Could you check a few things on this model? Use its own coordinates, in mm. A direction names the side the tool comes from. Coordinates: 2 decimals unless noted, no trailing zeros. Write each loop counter-clockwise with the first axis right and the second up, starting at its lowest first coordinate (ties: lowest second). Pieces come first, ordered by that corner, then holes.
Autodesk Inventor part; units mm, degrees
ref_plane "s1_XY" through (10.3124, 0, 0) normal (0, 0, 1) x (1, 0, 0)
ref_plane "s1_YZ" through (10.3124, 0, 0) normal (1, 0, 0) x (0, 1, 0)
ref_plane "s1_ZX" through (10.3124, 0, 0) normal (0, 1, 0) x (0, 0, 1)
sketch "Sketch_2" plane through (0, 0, 0) normal (0, 0, 1) x (1, 0, 0)
  line L0 (12.7, 0) -> (0, 0)
  line L1 (0, 0) -> (0, 7.098)
  line L2 (0, 7.098) -> (0.8395, 7.9375)
  line L3 (0.8395, 7.9375) -> (6.6726, 7.9375)
  line L4 (6.6726, 7.9375) -> (7.5121, 7.098)
  line L5 (7.5121, 7.098) -> (7.542, 7.0708)
  arc A0 (7.542, 7.0708) -> (8.1407, 6.839) centre (8.1407, 7.7279) ccw
  line L6 (8.1407, 6.839) -> (9.4234, 6.839)
  arc A1 (9.4234, 6.839) -> (10.3124, 7.7279) centre (9.4234, 7.7279) ccw
  line L7 (10.3124, 7.7279) -> (10.3124, 7.9057)
  line L8 (10.3124, 7.9057) -> (12.7, 7.9057)
  line L9 (12.7, 7.9057) -> (12.7, 0)
  line L10 (12.7, 0) -> (0, 0)
revolve "Revolution1" add sketch "Sketch_2" angle 360 about axis through (12.7, 0, 0) along (1, 0, 0)
thread "Thread1"
sketch "Sketch_3" plane through (0, 0, 0) normal (0, 0, 1) x (1, 0, 0)
  line L0 (41.275, 0) -> (12.7, 0)
  line L1 (12.7, 0) -> (12.7, 13.3731)
  line L2 (12.7, 13.3731) -> (13.462, 14.1351)
  line L3 (13.462, 14.1351) -> (34.8615, 14.1351)
  line L4 (34.8615, 14.1351) -> (34.8615, 12.846)
  line L5 (34.8615, 12.846) -> (35.6235, 12.846)
  line L6 (35.6235, 12.846) -> (36.3855, 13.6081)
  line L7 (36.3855, 13.6081) -> (40.513, 13.6081)
  line L8 (40.513, 13.6081) -> (41.275, 12.846)
  line L9 (41.275, 12.846) -> (41.275, 0)
  line L10 (41.275, 0) -> (12.7, 0)
revolve "Revolution2" add sketch "Sketch_3" angle 360 about axis through (41.275, 0, 0) along (1, 0, 0)
sketch "Sketch_5" plane through (0, 0, 0) normal (0, 0, 1) x (1, 0, 0)
  line L0 (41.275, 0) -> (0, 0)
  line L1 (0, 0) -> (0, 4.7752)
  line L2 (0, 4.7752) -> (0.762, 4.0132)
  line L3 (0.762, 4.0132) -> (41.275, 4.0132)
  line L4 (41.275, 4.0132) -> (41.275, 0)
  line L5 (41.275, 0) -> (0, 0)
revolve "Revolution3" cut sketch "Sketch_5" angle 360 about axis through (41.275, 0, 0) along (1, 0, 0)
sketch "Sketch_40" plane through (0, 0, 0) normal (0, 1, 0) x (-1, 0, 0)
  line L0 (-27.0002, 14.1351) -> (-27.0002, 0)
  line L1 (-27.0002, 0) -> (-30.1752, 0)
  line L2 (-30.1752, 0) -> (-30.1752, 3.8208)
  line L3 (-30.1752, 3.8208) -> (-31.5423, 4.6101)
  line L4 (-31.5423, 4.6101) -> (-31.8199, 13.5001)
  line L5 (-31.8199, 13.5001) -> (-32.4549, 14.1351)
  line L6 (-32.4549, 14.1351) -> (-27.0002, 14.1351)
  line L7 (-27.0002, 14.1351) -> (-27.0002, 0)
revolve "Revolution4" cut sketch "Sketch_40" angle 360 about axis through (27.0002, 0, 14.1351) along (0, 0, 1)
sketch "Sketch_47" plane through (0, 0, 0) normal (0, 0, 1) x (1, 0, 0)
  line L0 (35.6235, 0) -> (34.8615, 0)
  line L1 (34.8615, 12.5921) -> (35.6235, 12.5921)
  line L2 (35.6235, 12.5921) -> (35.6235, 12.846)
  line L3 (35.6235, 12.846) -> (35.2425, 12.846)
  line L4 (35.2425, 12.846) -> (34.984, 13.1046)
  arc A0 (34.984, 13.2842) -> (34.984, 13.1046) centre (35.0738, 13.1944) ccw
  line L5 (34.984, 13.2842) -> (35.7508, 14.0509)
  line L6 (35.7508, 14.0509) -> (35.7508, 14.1351)
  line L7 (35.7508, 14.1351) -> (35.5476, 14.1351)
  line L8 (35.5476, 14.1351) -> (34.8615, 13.449)
  line L9 (34.8615, 13.449) -> (34.8615, 12.5921)
revolve "Revolution5" add sketch "Sketch_47" angle 360 about axis through (35.6235, 0, 0) along (1, 0, 0)
ref_plane "s1_XY" through (10.3124, 0, 0) normal (0, 0, 1) x (1, 0, 0)
ref_plane "s1_YZ" through (10.3124, 0, 0) normal (1, 0, 0) x (0, 1, 0)
ref_plane "s1_ZX" through (10.3124, 0, 0) normal (0, 1, 0) x (0, 0, 1)
ref_plane "s2_XY" through (12.7, 0, 0) normal (0, 0, 1) x (1, 0, 0)
ref_plane "s2_YZ" through (12.7, 0, 0) normal (1, 0, 0) x (0, 1, 0)
ref_plane "s2_ZX" through (12.7, 0, 0) normal (0, 1, 0) x (0, 0, 1)
ref_plane "dp1_XY" through (12.7, 7.9057, 0) normal (0, 0, 1) x (1, 0, 0)
ref_plane "dp1_YZ" through (12.7, 7.9057, 0) normal (1, 0, 0) x (0, 1, 0)
ref_plane "dp1_ZX" through (12.7, 7.9057, 0) normal (0, 1, 0) x (0, 0, 1)
ref_plane "dp2_XY" through (12.7, -7.9057, 0) normal (0, 0, 1) x (1, 0, 0)
ref_plane "dp2_YZ" through (12.7, -7.9057, 0) normal (1, 0, 0) x (0, 1, 0)
ref_plane "dp2_ZX" through (12.7, -7.9057, 0) normal (0, 1, 0) x (0, 0, 1)
ref_plane "rod_guide_XY" through (0, 0, 0) normal (1, 0, 0) x (0, 0, -1)
ref_plane "rod_guide_YZ" through (0, 0, 0) normal (0, 0, -1) x (0, 1, 0)
ref_plane "rod_guide_ZX" through (0, 0, 0) normal (0, 1, 0) x (1, 0, 0)
ref_plane "to_tube_XY" through (35.6235, 0, 0) normal (1, 0, 0) x (0, 0, -1)
ref_plane "to_tube_YZ" through (35.6235, 0, 0) normal (0, 0, -1) x (0, 1, 0)
ref_plane "to_tube_ZX" through (35.6235, 0, 0) normal (0, 1, 0) x (1, 0, 0)
ref_plane "to_foot_bracket_XY" through (12.7, 0, 0) normal (1, 0, 0) x (0, 0, -1)
ref_plane "to_foot_bracket_YZ" through (12.7, 0, 0) normal (0, 0, -1) x (0, 1, 0)
ref_plane "to_foot_bracket_ZX" through (12.7, 0, 0) normal (0, 1, 0) x (1, 0, 0)
ref_plane "to_nut_XY" through (10.3124, 0, 0) normal (1, 0, 0) x (0, 0, -1)
ref_plane "to_nut_YZ" through (10.3124, 0, 0) normal (0, 0, -1) x (0, 1, 0)
ref_plane "to_nut_ZX" through (10.3124, 0, 0) normal (0, 1, 0) x (1, 0, 0)
ref_plane "to_trunnion_brackets_XY" through (18.2118, 0, 0) normal (0, 1, 0) x (1, 0, 0)
ref_plane "to_trunnion_brackets_YZ" through (18.2118, 0, 0) normal (1, 0, 0) x (0, 0, -1)
ref_plane "to_trunnion_brackets_ZX" through (18.2118, 0, 0) normal (0, 0, -1) x (0, 1, 0)
ref_plane "to_trunnion_brackets1_XY" through (18.2118, 15.875, 0) normal (0, 1, 0) x (1, 0, 0)
ref_plane "to_trunnion_brackets1_YZ" through (18.2118, 15.875, 0) normal (1, 0, 0) x (0, 0, -1)
ref_plane "to_trunnion_brackets1_ZX" through (18.2118, 15.875, 0) normal (0, 0, -1) x (0, 1, 0)
ref_plane "to_trunnion_brackets2_XY" through (18.2118, -15.875, 0) normal (0, 1, 0) x (1, 0, 0)
ref_plane "to_trunnion_brackets2_YZ" through (18.2118, -15.875, 0) normal (1, 0, 0) x (0, 0, -1)
ref_plane "to_trunnion_brackets2_ZX" through (18.2118, -15.875, 0) normal (0, 0, -1) x (0, 1, 0)
ref_plane "t111_XY" through (12.7, 0, 0) normal (1, 0, 0) x (0, 0, -1)
ref_plane "t111_YZ" through (12.7, 0, 0) normal (0, 0, -1) x (0, 1, 0)
ref_plane "t111_ZX" through (12.7, 0, 0) normal (0, 1, 0) x (1, 0, 0)
ref_plane "t1_XY" through (12.7, 0, 0) normal (1, 0, 0) x (0, 0, -1)
ref_plane "t1_YZ" through (12.7, 0, 0) normal (0, 0, -1) x (0, 1, 0)
ref_plane "t1_ZX" through (12.7, 0, 0) normal (0, 1, 0) x (1, 0, 0)
ref_plane "port_XY" through (27.0002, 0, 0) normal (0, 0, 1) x (1, 0, 0)
ref_plane "port_YZ" through (27.0002, 0, 0) normal (1, 0, 0) x (0, 1, 0)
ref_plane "port_ZX" through (27.0002, 0, 0) normal (0, 1, 0) x (0, 0, 1)
ref_plane "to_screw_XY" through (27.0002, 10.2743, -7.0485) normal (0, 1, 0) x (1, 0, 0)
ref_plane "to_screw_YZ" through (27.0002, 10.2743, -7.0485) normal (1, 0, 0) x (0, 0, -1)
ref_plane "to_screw_ZX" through (27.0002, 10.2743, -7.0485) normal (0, 0, -1) x (0, 1, 0)
properties part number "09R000_rod_guide"
Item 1: Will these pins go through, and if not, where does the flat tip stop? pin 1 Ø10 at (x, y) = (6, 3.5) entering from -Z; pin 2 Ø12 at (x, y) = (33.5, -10.5) entering from +Z; pin 3 Ø4 at (x, y) = (25.5, 5) entering from -Z.
Item 2: I want a section at B-B, the plane y = 0. Count the separate pieces of the cut face and the enclosed holes in it, then the cut area to 3 significant figures.
Item 3: I want a section at C-C, the plane x = 4. List the corners of the cut face in (y, z) for me (1 decimal), then the cut area to 3 significant figures.
Item 4: If I drill on line 1 along Z through (x, y) = (12, 0); line 2 along Z through (x, y) = (20, 0); line 3 along X through (y, z) = (-2.25, 6.75) (3 decimals), over which ranges is the centre line in solid material (lowest first)?
Item 5: Which directions (+Z, -Z, +X, -X, +Y, -Y) give clear straight access to the entire face, cutting with the end or side of a thin tool? Please do faces 1 (the conical face through (23.549, 3.165, 9.117)), 2 (the cylindrical face through (38.48, -10.8, -8.28)), 3 (the cylindrical face through (8.791, 6.523, 2.054)).
Item 6: If we mould it in two halves opening along X, with no side actions, what happens to faces 4 (the cylindrical face through (26.948, -3.175, 3.299)), 5 (the cylindrical face through (3.8, -1.72, -7.75))? For each: released by +X, released by -X, zero draft, split by the parting line, or undercut.
Item 7: I want a section at A-A, the plane x = 37. List the corners of the cut face in (y, z) for me, then the cut area to 3 significant figures.
Taken from the geometry:
1. pin 1: stops at z = -7.94
1. pin 2: stops at z = 13.4
1. pin 3: stops at z = -13.81
2. separate pieces: 3
2. enclosed holes: 0
2. area: 567 mm2
3. outline: circle Ø15.9 at (0, 0); hole circle Ø8 at (0, 0)
3. area: 147 mm2
4. line 1: z = -7.91 to -4.01, 4.01 to 7.91
4. line 2: z = -14.14 to -4.01, 4.01 to 14.14
4. line 3: x = 0.017 to 7.495, 10.067 to 22.978, 31.023 to 41.275
5. face 1: +Z
5. face 2: +X
5. face 3: none
6. face 4: undercut
6. face 5: zero draft
7. outline: circle Ø27.22 at (0, 0); hole circle Ø8.03 at (0, 0)
7. area: 531 mm2
